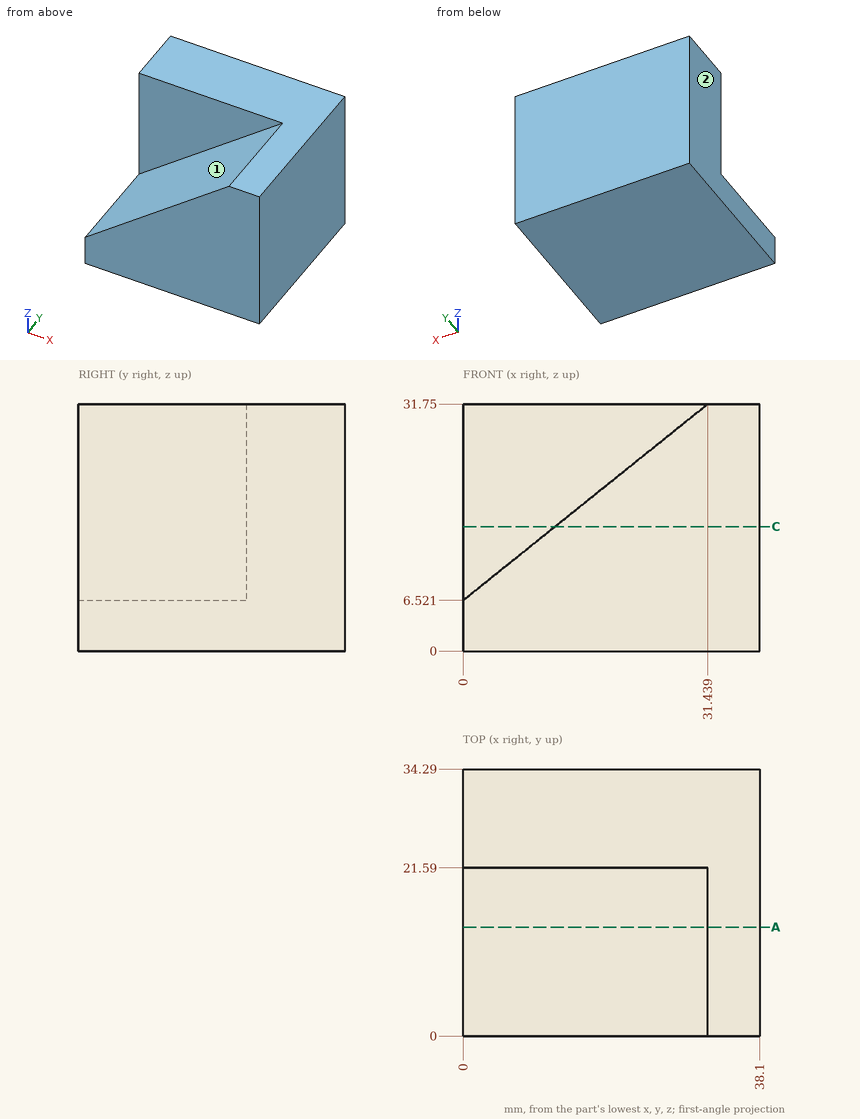
For this review, use the dimensioned drawing (mm, ordinates from the lowest corner) and the shaded views. A direction names the side the tool comes from. Round coordinates to 2 decimals unless told otherwise and drop trailing zeros. Write each loop counter-clockwise with the first axis right and the second up, starting at its lowest first coordinate (ties: lowest second). Pieces come first, ordered by that corner, then holes. Notation, with made-up numbers: (44, -2.75) - (98, -2.75) arc R31 ccw to (98, 31.25) - close; hole circle Ø4 at (-22.5, 7.5). An arc over 180 degrees is marked (long way). One line per item, written item: value. Start each with the question number.
1. Consider section A-A on y = 14. Write out the cut boundary in (x, z).
2. Consider section C-C on z = 16. Write out the cut boundary in (x, y), and give its area (3 significant figures).
3. To check wall thickness, follow L1, parallel to Y at x = 8, z = 21; L2, parallel to X at y = 6.5, z = 22; L3, parallel to Z at x = 23, y = 12. State the ranges of each line that lie inside material, in increasing order. Write a range as from..to.
4. Machinability: for the marked faces 1 and 2, which of the approach directions +Z, -Z, +X, -X, +Y, -Y give a long, thin tool a straight path to every point of the face, cutting with its end or side? Answer none if there is none.
5. Clearance check with flat-ended pins moving along their axes: P1, Ø6, axis at x = 12, z = 28, coming from the -Y side; P2, Ø12, axis at y = 12.5, z = 3.5, coming from the -X side; P3, Ø3, axis at y = 19.5, z = 13, coming from the -X side (1 decimal). State where each tip first meets the part, or that it passes through.
Checks:
1. outline: (0, 0) - (38.1, 0) - (38.1, 31.75) - (31.44, 31.75) - (0, 6.52) - close
2. outline: (0, 21.59) - (11.81, 21.59) - (11.81, 0) - (38.1, 0) - (38.1, 34.29) - (0, 34.29) - close
2. area: 1,050 mm^2
3. L1: y = 21.59..34.29
3. L2: x = 19.29..38.1
3. L3: z = 0..24.98
4. face 1: +Z, -X, -Y
4. face 2: +Z, -Z, -X, +Y, -Y
5. P1: stops at y = 21.59
5. P2: stops at x = 0
5. P3: stops at x = 6.2
